Study the drawing (mm; zero at the part's minimum x, y, z) and answer. A direction names the side the tool comes from. Coordinates: 2 decimals unless noted, no trailing zeros. Order: outer loops, then holes, each group sorted by start corner. A loop starts at its lowest first (then second) coordinate and runs counter-clockwise, first axis right, second up.
1. Flat-ended cylindrical pins translate along their axes: pin 1 Ø10 at (y, z) = (139, 51.5) entering from -X; pin 2 Ø5 at (x, z) = (80.5, 57.5) entering from -Y; pin 3 Ø2 at (x, y) = (56, 46) entering from -Z (1 decimal); pin 4 Ø12 at (y, z) = (75, 43.5) entering from -X. Find the tip coordinate at first contact, or state that the pin passes through.
2. The part is cut by section D-D, the plane y = 61. Give the vertices of the cut face in (x, z).
3. The part is cut by section B-B, the plane z = 100.5. Give the vertices of the cut face in (x, y).
4. The part is cut by section A-A, the plane y = 144. Give the vertices of the cut face in (x, z) (1 decimal), then the cut area to 3 significant figures.
5. Find the intervals of material crossed by probe 1 along Y at (x, z) = (64, 96); probe 2 along Z at (x, y) = (45.5, 98.5); probe 3 along X at (y, z) = (39.5, 52.5) (1 decimal), in increasing order.
6. The part is cut by section C-C, the plane x = 9. Give the vertices of the cut face in (y, z).
7. A tool of negligible diameter and unlimited length cuts with its end or side. For the marked faces 1 and 2, from which of +Z, -Z, +X, -X, +Y, -Y can it reach the whole face along a straight path? Write none if from no direction.
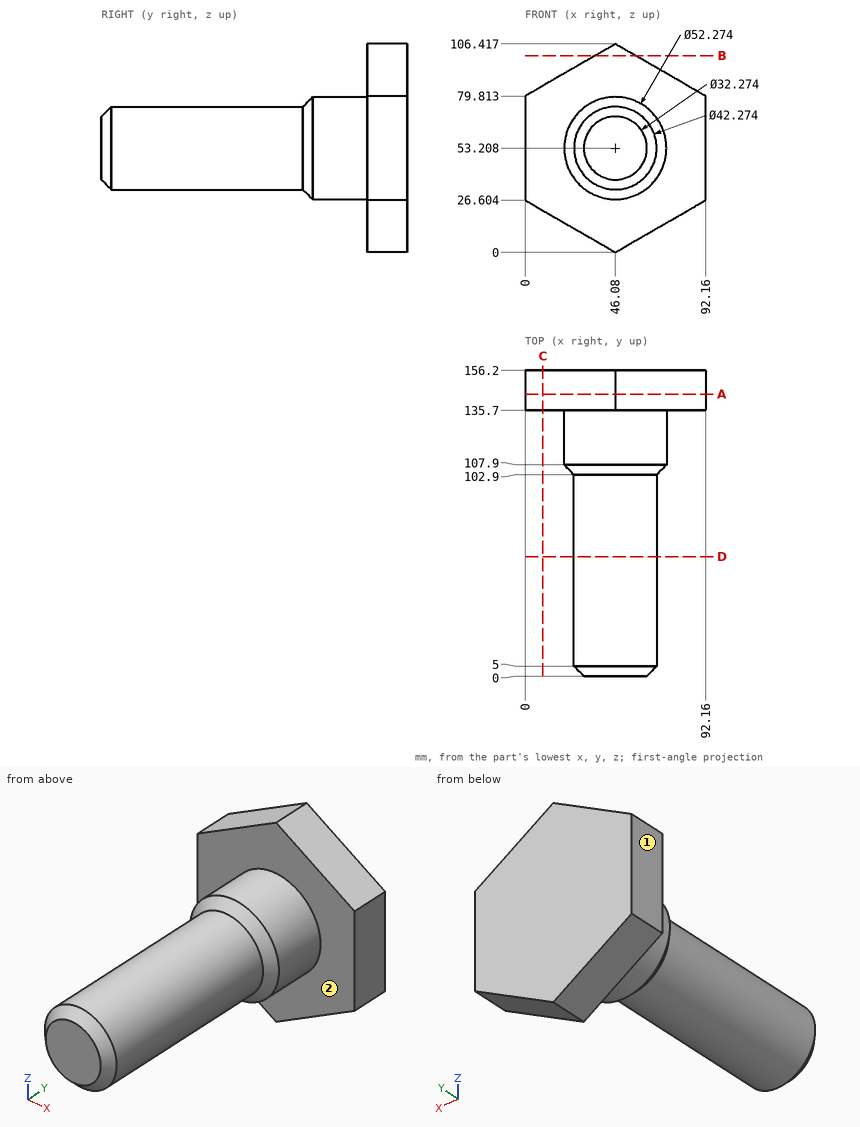
Geometry says:
1. pin 1: stops at x = 0
1. pin 2: stops at y = 135.7
1. pin 3: stops at z = 34
1. pin 4: stops at x = 25.27
2. outline: circle Ø42.27 at (46.08, 53.21)
3. outline: (35.83, 135.7) - (56.33, 135.7) - (56.33, 156.2) - (35.83, 156.2) - close
4. outline: (0, 26.6) - (46.1, 0) - (92.2, 26.6) - (92.2, 79.8) - (46.1, 106.4) - (0, 79.8) - close
4. area: 7,360 mm2
5. probe 1: y = 135.7 to 156.2
5. probe 2: z = 32.08 to 74.34
5. probe 3: x = 25 to 67.2
6. outline: (135.7, 21.41) - (156.2, 21.41) - (156.2, 85.01) - (135.7, 85.01) - close
7. face 1: +Z, -Z, -X, +Y, -Y
7. face 2: -Y
